The listing builds one solid part. Answer for the finished solid, in the listing's coordinates (mm). Face numbers are marked on the shaded views. A direction names the side the tool comes from. Round coordinates to 2 decimals unless told otherwise and drop trailing zeros. Write each loop counter-clockwise with the first axis right and the second up, starting at its lowest first coordinate (ties: lowest second). Pieces come first, ordered by that corner, then holes.
Item 1: Find section D-D on x = -1.75. Give the vertices of the cut face in (y, z), then the cut area to 3 significant figures.
Item 2: Find section B-B on x = -8. Give the vertices of the cut face in (y, z).
Item 3: A tool of negligible diameter and unlimited length cuts with its end or side. For the marked faces 1 and 2, from which of +Z, -Z, +X, -X, +Y, -Y can it reach the whole face along a straight path? Write none if from no direction.
Item 4: For a pull along X with two mould halves and no side action, classify the marked faces 3, 4, 5 and 6 as +X half, -X half, draft (parallel to the pull), parting line (faces both ways), or undercut.
Item 5: Find the intervals of material crossed by probe 1 along Y at (x, z) = (8, 2.55); probe 2 along X at (y, z) = (-0.25, 1); probe 3 along X at (y, z) = (-0.5, 0.8), in increasing order.
Item 6: Each of these flat-tipped pins is pushed along its axis until it touches: pin 1 (1.5 mm diameter, centred on y = 2, z = 1, fed in from +X); pin 2 (0.5 mm diameter, centred on y = 0.5, z = 1, fed in from -X); pin 3 (1.3 mm diameter, centred on y = 1, z = 0.5, fed in from +X); pin 4 (1.6 mm diameter, centred on x = 8, y = 0, fed in from -Z) (3 decimals). Where does it stop, or does it pass through?
Item 7: Find section A-A on z = 0.65. Give the number of separate pieces and of enclosed holes in the cut face, then the cut area to 3 significant figures.
```python
from build123d import *

# Parameters (mm, degrees)
SKETCH1_W           = 24
SKETCH1_H           = 6
SKETCH1_R           = 1.3
BOSS_EXTRUDE1_DEPTH = 3.2
SKETCH2_W           = 5.5
SKETCH2_H           = 6
CUT_EXTRUDE1_DEPTH  = 1.6
FILLET1_R           = 3
FILLET2_R           = 0.5


with BuildPart() as part:
    # Sketch1 → Boss-Extrude1 (new body)
    with BuildSketch(Plane.XY):
        Rectangle(SKETCH1_W, SKETCH1_H)
        with Locations((-8, 0)):
            Circle(SKETCH1_R, mode=Mode.SUBTRACT)
        with Locations((8, 0)):
            Circle(SKETCH1_R, mode=Mode.SUBTRACT)
    extrude(amount=BOSS_EXTRUDE1_DEPTH)

    # Sketch2 → Cut-Extrude1 (cut)
    with BuildSketch(Plane(origin=(0, 0, 0), x_dir=(-1, 0, 0), z_dir=(0, 0, -1))):
        Rectangle(SKETCH2_W, SKETCH2_H)
    extrude(amount=-CUT_EXTRUDE1_DEPTH, mode=Mode.SUBTRACT)

    # Fillet1
    fillet1_edges = [part.edges().sort_by_distance(p)[0] for p in [
        (-12, -3, 1.6),
        (-12, 3, 1.6),
        (12, -3, 1.6),
        (12, 3, 1.6),
    ]]
    fillet(fillet1_edges, radius=FILLET1_R - 0.0001)  # a hair under: the kernel refuses the full size

    # Fillet2
    fillet2_edges = [part.edges().sort_by_distance(p)[0] for p in [
        (-2.75, 3, 0.8),
        (0, -3, 1.6),
        (-2.75, -3, 0.8),
        (2.75, -3, 0.8),
        (0, 3, 1.6),
        (2.75, 3, 0.8),
        (0, -3, 3.2),
        (0, 3, 3.2),
        (11.121349633, 2.121349633, 3.2),
        (11.121349633, -2.121349633, 3.2),
        (-11.121349633, 2.121349633, 3.2),
        (-11.121349633, -2.121349633, 3.2),
    ]]
    fillet(fillet2_edges, radius=FILLET2_R)


solid = part.part
```
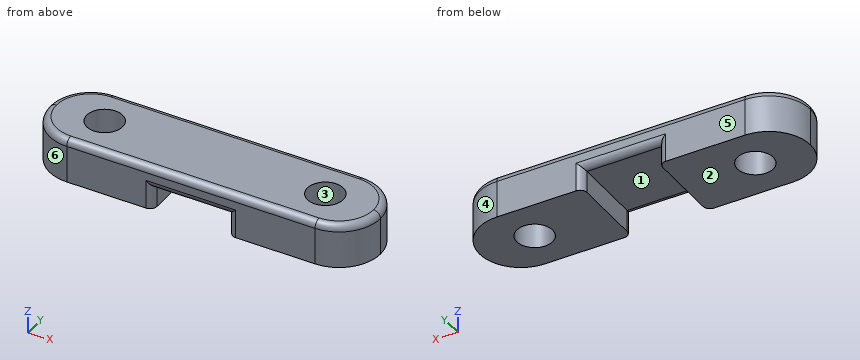
Check values:
1. outline: (-3, 2.1) arc R0.5 ccw to (-2.5, 1.6) - (2.5, 1.6) arc R0.5 ccw to (3, 2.1) - (3, 2.7) arc R0.5 ccw to (2.5, 3.2) - (-2.5, 3.2) arc R0.5 ccw to (-3, 2.7) - close
1. area: 9.39 mm2
2. outline: (-3, 0) - (-1.3, 0) - (-1.3, 3.2) - (-2.5, 3.2) arc R0.5 ccw to (-3, 2.7) - close; (1.3, 0) - (3, 0) - (3, 2.7) arc R0.5 ccw to (2.5, 3.2) - (1.3, 3.2) - close
3. face 1: -Z, +Y, -Y
3. face 2: -Z, +X, -X, +Y, -Y
4. face 3: undercut
4. face 4: +X half
4. face 5: draft
4. face 6: -X half
5. probe 1: y = -3 to -1.3, 1.3 to 3
5. probe 2: x = -11.99 to -9.28, -6.72 to -2.75, 2.75 to 6.72, 9.28 to 11.99
5. probe 3: x = -11.96 to -9.2, -6.8 to -2.75, 2.75 to 6.8, 9.2 to 11.96
6. pin 1: stops at x = 11.73
6. pin 2: stops at x = -11.99
6. pin 3: stops at x = 11.98
6. pin 4: passes through
7. separate pieces: 2
7. enclosed holes: 2
7. area: 92.4 mm2
